Could you check a few things on this model? Use its own coordinates, in mm. A direction names the side the tool comes from. Give positions to 0.01 mm unless a question says otherwise; leave off trailing zeros. Loops run counter-clockwise (first coordinate to the right, second up) from the corner with the lowest first, then second, coordinate; pieces in that order, holes last.
1. Imagine slicing it at C-C (z = 0.5). List the corners of the cut face in (x, y) for me, plus the area to 3 significant figures.
2. For P1, Ø7, axis at x = -10, y = 14, coming from the -Z side; P2, Ø1.6, axis at x = 8, y = 7.5, coming from the -Z side; P3, Ø6.5, axis at y = 14, z = -43.5, coming from the +X side; P4, Ø7.5, axis at x = -19.66, z = -35.02, coming from the -Y side, each with a flat end and sliding along its axis, tell me the tip position at first contact or that it passes through.
3. Imagine slicing it at A-A (z = -14.5). List the corners of the cut face in (x, y) for me.
4. For faces 1 (the cylindrical face through (0.33, 8.17, 6.23)), 2 (the cylindrical face through (-28.289, 10.14, 11.226)), 3 (the flat face through (-8, 10, -36.338)), which set-ups out of +Z, -Z, +X, -X, +Y, -Y let a thin tool reach every point of the face, with its end or its side?
5. Imagine slicing it at B-B (x = 28.5). List the corners of the cut face in (y, z) for me, plus the area to 3 significant figures.
6. Imagine slicing it at D-D (x = 3.5). List the corners of the cut face in (y, z) for me.
7. I need wall thicknesses on line 1 along Y through (x, z) = (0, -13.75); line 2 along X through (y, z) = (1.75, -12); line 3 along Z through (x, y) = (2, 4). Which ranges of each line are inside material? Lowest first, please.
```python
from build123d import *

# Parameters (mm, degrees)
SKETCH1_R                  = 4.125
BOSS_EXTRUDE1_DEPTH        = 20
FILLET2_R                  = 5
FILLET3_R                  = 5
FILLET4_R                  = 6
FILLET5_R                  = 6
FILLET6_R                  = 2
FILLET7_R                  = 3
FILLET10_R                 = 2
UPPER_VERTEX_HOLES_D       = 3
UPPER_VERTEX_HOLES_DEPTH   = 30
UPPER_VERTEX_HOLES_TIP     = 0.901290929
F_8_0_199_DIAMETER_HOLE2_D = 4
F_8_0_199_DIAMETER_HOLE3_D = 4
SKETCH12_W                 = 2
SKETCH12_H                 = 41.945563192
SKETCH16_W                 = 2
SKETCH16_H                 = 41.945563192


with BuildPart() as part:
    # Sketch1 → Boss-Extrude1 (new body)
    with BuildSketch(Plane(origin=(0, 0, 0), x_dir=(1, 0, 0), z_dir=(0, 1, 0))):
        with BuildLine():
            Line((-28.643593539, -10.537386441), (-38.169872981, -27.037386441))
            Line((-38.169872981, -27.037386441), (-42.5, -24.537386441))
            Line((-42.5, -24.537386441), (-14.5, 23.960036171))
            Line((-14.5, 23.960036171), (-31.820508076, 33.960036171))
            ThreePointArc((-31.820508076, 33.960036171), (0, 50.621689136), (31.820508076, 33.960036171))
            Line((31.820508076, 33.960036171), (14.5, 23.960036171))
            Line((14.5, 23.960036171), (42.5, -24.537386441))
            Line((42.5, -24.537386441), (38.169872981, -27.037386441))
            Line((38.169872981, -27.037386441), (28.643593539, -10.537386441))
            Line((28.643593539, -10.537386441), (-28.643593539, -10.537386441))
        make_face()
        with Locations((19.660254038, 35.022213998)):
            Circle(SKETCH1_R, mode=Mode.SUBTRACT)
        with Locations((-19.660254038, 35.022213998)):
            Circle(SKETCH1_R, mode=Mode.SUBTRACT)
        Polygon((-12.0447733, 18.212613559), (-26.47853003, -6.787386441), (-7.5, -6.787386441), (-3.75, -2.037386441), (3.75, -2.037386441), (7.5, -6.787386441), (26.47853003, -6.787386441), (12.0447733, 18.212613559), (3.75, 10.462613559), (-3.75, 10.462613559), align=None, mode=Mode.SUBTRACT)
        Polygon((-9.999491924, 47.962613559), (10.000508076, 47.962613559), (10.000508076, 39.587613559), (6.750508076, 39.587613559), (6.750508076, 36.337613559), (10.000508076, 36.337613559), (10.000508076, 27.962613559), (-9.999491924, 27.962613559), (-9.999491924, 36.337613559), (-6.749491924, 36.337613559), (-6.749491924, 39.587613559), (-9.999491924, 39.587613559), align=None, mode=Mode.SUBTRACT)
    extrude(amount=BOSS_EXTRUDE1_DEPTH)

    # Fillet2
    fillet2_edges = [part.edges().sort_by_distance(p)[0] for p in [
        (-28.643593539, 10, 10.537386441),
    ]]
    fillet(fillet2_edges, radius=FILLET2_R)

    # Fillet3
    fillet3_edges = [part.edges().sort_by_distance(p)[0] for p in [
        (28.643593539, 10, 10.537386441),
    ]]
    fillet(fillet3_edges, radius=FILLET3_R)

    # Fillet4
    fillet4_edges = [part.edges().sort_by_distance(p)[0] for p in [
        (-26.47853003, 10, 6.787386441),
    ]]
    fillet(fillet4_edges, radius=FILLET4_R)

    # Fillet5
    fillet5_edges = [part.edges().sort_by_distance(p)[0] for p in [
        (26.47853003, 10, 6.787386441),
    ]]
    fillet(fillet5_edges, radius=FILLET5_R)

    # Fillet6
    fillet6_edges = [part.edges().sort_by_distance(p)[0] for p in [
        (-12.0447733, 10, -18.212613559),
        (12.0447733, 10, -18.212613559),
    ]]
    fillet(fillet6_edges, radius=FILLET6_R)

    # Fillet7
    fillet7_edges = [part.edges().sort_by_distance(p)[0] for p in [
        (-3.75, 10, -10.462613559),
        (-3.75, 10, 2.037386441),
        (3.75, 10, 2.037386441),
        (3.75, 10, -10.462613559),
    ]]
    fillet(fillet7_edges, radius=FILLET7_R)

    # Fillet10
    fillet10_edges = [part.edges().sort_by_distance(p)[0] for p in [
        (-38.169872981, 10, 27.037386441),
        (-42.5, 10, 24.537386441),
        (42.5, 10, 24.537386441),
        (38.169872981, 10, 27.037386441),
    ]]
    fillet(fillet10_edges, radius=FILLET10_R)

    # Upper Vertex Holes
    with Locations(Plane.XY.offset(10.537386441)):
        with Locations((0, 9.632614612)):
            Hole(UPPER_VERTEX_HOLES_D / 2, depth=UPPER_VERTEX_HOLES_DEPTH)
            with Locations((0, 0, -(UPPER_VERTEX_HOLES_DEPTH + UPPER_VERTEX_HOLES_TIP / 2))):  # 118° drill point
                Cone(0, UPPER_VERTEX_HOLES_D / 2, UPPER_VERTEX_HOLES_TIP, mode=Mode.SUBTRACT)

    # #8 (0.199) Diameter Hole2 (through all)
    with Locations(Plane(origin=(16.919872981, 0, -9.76869322), x_dir=(0.5, 0, 0.866025404), z_dir=(-0.866025404, 0, 0.5))):
        with Locations((33.417096231, 10)):
            Hole(F_8_0_199_DIAMETER_HOLE2_D / 2)

    # #8 (0.199) Diameter Hole3 (through all)
    with Locations(Plane(origin=(-16.919872981, 0, -9.76869322), x_dir=(0.5, 0, -0.866025404), z_dir=(0.866025404, 0, 0.5))):
        with Locations((-33.417096231, 10)):
            Hole(F_8_0_199_DIAMETER_HOLE3_D / 2)

    # Sketch12 → #8 (0.199) Diameter Hole5 (revolve, cut)
    with BuildSketch(Plane(origin=(17.292785365, 10, -9.122790024), x_dir=(0.5, 0, 0.866025404), z_dir=(0, 1, 0))):
        with Locations((1, 20.972781596)):
            Rectangle(SKETCH12_W, SKETCH12_H)
    revolve(axis=Axis((11.793524051, 10, -5.947790024), (0.866025404, 0, -0.5)), mode=Mode.SUBTRACT)

    # Sketch16 → #8 (0.199) Diameter Hole6 (revolve, cut)
    with BuildSketch(Plane(origin=(-17.292785365, 10, -9.122790024), x_dir=(0.5, 0, -0.866025404), z_dir=(0, 1, 0))):
        with Locations((1, 20.972781596)):
            Rectangle(SKETCH16_W, SKETCH16_H)
    revolve(axis=Axis((-11.793524051, 10, -5.947790024), (-0.866025404, 0, -0.5)), mode=Mode.SUBTRACT)

    # Sketch18 → #8 (0.199) Diameter Hole7 (revolve, cut)
    with BuildSketch(Plane(origin=(0.000508076, 10, -47.962613559), x_dir=(0, -1, 0), z_dir=(1, 0, 0))):
        Polygon((0, 0), (0, 31.2017212), (1.999999937, 30), (1.999999937, 0), align=None)
    revolve(axis=Axis((0.000508076, 10, -41.612613559), (0, 0, -1)), mode=Mode.SUBTRACT)


solid = part.part
```
Derived:
1. outline: (-28.62, 0) - (-22.08, 0) - (-22.08, 20) - (-28.62, 20) - close; (22.08, 0) - (28.62, 0) - (28.62, 20) - (22.08, 20) - close
1. area: 262 mm2
2. P1: stops at z = -50.07
2. P2: stops at z = -49.95
2. P3: stops at x = 26.37
2. P4: passes through
3. outline: (-19.96, 0) - (-14.19, 0) - (-14.19, 20) - (-19.96, 20) - close; (-8.07, 0) - (8.07, 0) - (8.07, 20) - (-8.07, 20) - close; (14.19, 0) - (19.96, 0) - (19.96, 20) - (14.19, 20) - close; hole circle Ø3 at (0, 9.63)
4. face 1: +Z
4. face 2: +Z, +Y, -Y
4. face 3: +Y, -Y
5. outline: (0, -38.11) - (20, -38.11) - (20, -32.04) - (0, -32.04) - close; (0, 0.29) - (20, 0.29) - (20, 11.36) - (0, 11.36) - close
5. area: 343 mm2
6. outline: (0, -50.46) - (20, -50.46) - (20, -47.96) - (0, -47.96) - close; (0, -27.96) - (20, -27.96) - (20, -10.61) - (0, -10.61) - close; (0, 2.29) - (20, 2.29) - (20, 10.54) - (0, 10.54) - close
7. line 1: y = 0 to 8.13, 11.13 to 20
7. line 2: x = -21.41 to -15.63, -5.4 to 5.4, 15.63 to 21.41
7. line 3: z = -50.57 to -47.96, -27.96 to -10.46, 2.04 to 10.54
